Model file for the job. Use its own axes, mm. A direction names the side the tool comes from. Give positions to 0.01 mm unless a question says otherwise; leave off trailing zeros. Order: outer loops, then holes, each group sorted by start corner. A loop starts at its lowest first (then second) coordinate and runs counter-clockwise, first axis right, second up. Notation, with made-up numbers: M -12.5,-15 L 4.5,-15 A14 ccw 4.5,6 Z; hole C 69.5,32.5 d11. An arc over 180 degrees is marked long. Return JSON: item names as keys, results as strings. Group by question number.
1. Slice it at A-A on x = 8. List the corners of the cut face in (y, z), then the cut area to 3 significant figures.
2. Slice it at C-C on y = -5. List the corners of the cut face in (x, z).
3. Pin check, flat tips, straight feed: pin 1 (10 mm diameter, centred on x = -4.5, z = 40, fed in from +Y); pin 2 (3 mm diameter, centred on x = -7.5, z = -39.5, fed in from +Y); pin 3 (8.5 mm diameter, centred on x = -2.5, z = -82.5, fed in from -Y); pin 4 (4 mm diameter, centred on x = -9, z = -42, fed in from +Y). Stop position of each tip, or through.
4. Wall check: probe 1 along Z at (x, y) = (0, 23.25) (3 decimals); probe 2 along Y at (x, z) = (4, 71); probe 3 along X at (y, z) = (21.5, 69.85) (3 decimals). Give the ranges that are in metal, low to high. Write a range as [from, to].
5. 3-axis set-ups, long thin cutter, end or side, ignore diameter. For faces 1 (the face through (10.16, -7, 20)), 2 (the face through (13, -7.62, -39)), 3 (the face through (0, -10.16, -84)), 4 (the face through (-13, 0, -4)): which of +Z, -Z, +X, -X, +Y, -Y reach the whole face in a straight line?
6. Slice it at B-B on z = -35.5. List the corners of the cut face in (x, y), then the cut area to 3 significant figures.
7. Two-plate mould, pull along X, no slides. Class faces 5 (the face through (-15.24, -4, 23)), 6 (the face through (-13, -7.62, -39)), 7 (the face through (0, -16.51, 51)): released by +X, released by -X, zero draft, split by the parting line, or undercut.
8. Slice it at D-D on z = 49. List the corners of the cut face in (x, y), then the cut area to 3 significant figures.
from build123d import *

# Parameters (mm, degrees)
F1_DEPTH     = 16.51
F2_W         = 8.89
F2_H         = 106.68
F3_DEPTH     = 50.8
F4_W         = 5.08
F4_H         = 63.5
F4_W_2       = 25.4
F5_DEPTH     = 5.08
F6_T1_DEPTH  = 5.08
F6_T6_DEPTH  = 43.0474778593
F6_T12_DEPTH = 81.0149557187
F8_DEPTH     = 25.4
F9_W         = 20.32
F9_H         = 15.2493301511
F10_DEPTH    = 2.54
F11_W        = 20.32
F11_H        = 2.54
F12_DEPTH    = 2.54
F13_R        = 0.635
F14_DEPTH    = 2.54
F15_W        = 10.16
F15_H        = 10.16
F15_R        = 0.635
F16_DEPTH    = 1.27


# Not quite as in the source:
# - a fillet or chamfer that OpenCascade refuses, or shapes differently, is made with other operations: its cross-section is extruded or revolved along the edge and cut away or added


with BuildPart() as f1:
    # F0 (on Front) → F1 (new body)
    with BuildSketch(Plane.XZ):
        Polygon((15.24, 6.35), (15.24, 82.55), (10.16, 82.55), (10.16, -82.55), (-10.16, -82.55), (-10.16, 82.55), (-15.24, 82.55), (-15.24, 6.35), (-15.24, -87.63), (15.24, -87.63), align=None)
    extrude(amount=F1_DEPTH)

    # F2 (on face) → F3 (cut)
    with BuildSketch(Plane(origin=(-15.24, 0, 0), x_dir=(0, -1, 0), z_dir=(-1, 0, 0))):
        with Locations((12.065, -34.29)):
            Rectangle(F2_W, F2_H)
    extrude(amount=-F3_DEPTH, mode=Mode.SUBTRACT)

    # F4 (on face) → F5 (join)
    with BuildSketch(Plane.XZ.offset(16.51)):
        with Locations((-12.7, 50.8)):
            Rectangle(F4_W, F4_H)
        with Locations((2.54, 50.8)):
            Rectangle(F4_W_2, F4_H)
    extrude(amount=F5_DEPTH)

    # F6: fillet of radius 15.24 on 1 edges, made by hand

    # F6_s2 → F6_t1 (join)
    with BuildSketch(Plane.YZ.offset(-15.24)):
        with BuildLine():
            ThreePointArc((-21.59, 19.05), (-11.6436636998, 14.1805376301), (-7.62, 3.8630088563))
            Line((-7.62, 3.8630088563), (-7.62, 19.05))
            Line((-7.62, 19.05), (-21.59, 19.05))
        make_face()
    extrude(amount=F6_T1_DEPTH)


with BuildPart() as f6_tool4:
    # F6_s5 → F6_t6 (new body)
    with BuildSketch(Plane.YZ.offset(-15.24)):
        with BuildLine():
            ThreePointArc((-21.59, 19.05), (-11.6436636998, 14.1805376301), (-7.62, 3.8630088563))
            Line((-7.62, 3.8630088563), (-7.62, 19.05))
            Line((-7.62, 19.05), (-21.59, 19.05))
        make_face()
    extrude(amount=F6_T6_DEPTH)

    split(bisect_by=Plane.YZ.offset(15.24), keep=Keep.BOTTOM)

    split(bisect_by=Plane.XZ.offset(16.51), keep=Keep.TOP)


with BuildPart() as f1_1:
    add(f1.part)

    # F6_t3: union F6_tool4
    add(f6_tool4.part)


with BuildPart() as f6_tool10:
    # F6_s11 → F6_t12 (new body)
    with BuildSketch(Plane.YZ.offset(-53.2074778593)):
        with BuildLine():
            ThreePointArc((-21.59, 19.05), (-11.6436636998, 14.1805376301), (-7.62, 3.8630088563))
            Line((-7.62, 3.8630088563), (-7.62, 19.05))
            Line((-7.62, 19.05), (-21.59, 19.05))
        make_face()
    extrude(amount=F6_T12_DEPTH)

    split(bisect_by=Plane.YZ.offset(15.24), keep=Keep.BOTTOM)

    split(bisect_by=Plane.YZ.offset(10.16), keep=Keep.TOP)


with BuildPart() as f1_2:
    add(f1_1.part)

    # F6_t9: union F6_tool10
    add(f6_tool10.part)

    # F7 (on face) → F8 (join)
    with BuildSketch(Plane.XY.offset(82.55)):
        Polygon((10.16, 0), (15.24, 0), (15.24, 22.86), (-15.24, 22.86), (-15.24, 0), (-10.16, 0), align=None)
    extrude(amount=-F8_DEPTH)

    # F9 (on face) → F10 (join)
    with BuildSketch(Plane(origin=(0, 0, 0), x_dir=(-1, 0, 0), z_dir=(0, 1, 0))):
        Polygon((-15.24, -67.3006698489), (-15.24, -87.63), (15.24, -87.63), (15.24, -67.3006698489), (10.16, -67.3006698489), (10.16, -82.55), (-10.16, -82.55), (-10.16, -67.3006698489), align=None)
        with Locations((0, -74.9253349245)):
            Rectangle(F9_W, F9_H)
    extrude(amount=F10_DEPTH)

    # F11 (on face) → F12 (join)
    with BuildSketch(Plane.XZ.offset(7.62)):
        with Locations((0, -81.28)):
            Rectangle(F11_W, F11_H)
        Polygon((-15.24, -80.01), (-15.24, -87.63), (15.24, -87.63), (15.24, -80.01), (10.16, -80.01), (10.16, -82.55), (-10.16, -82.55), (-10.16, -80.01), align=None)
    extrude(amount=F12_DEPTH)

    # F13 (on face) → F14 (cut)
    with BuildSketch(Plane(origin=(0, 22.86, 0), x_dir=(-1, 0, 0), z_dir=(0, 1, 0))):
        with Locations((0, 69.85)):
            Circle(F13_R)
    extrude(amount=-F14_DEPTH, mode=Mode.SUBTRACT)

    # F15 (on face) → F16 (join)
    with BuildSketch(Plane(origin=(0, 22.86, 0), x_dir=(-1, 0, 0), z_dir=(0, 1, 0))):
        with Locations((0, 69.85)):
            Rectangle(F15_W, F15_H)
        with Locations((0, 69.85)):
            Circle(F15_R, mode=Mode.SUBTRACT)
    extrude(amount=F16_DEPTH)


solid = f1_2.part
Result:
{
 "1": {"outline": "M -21.59,19.05 A15.24 cw -16.51,17.72 L -16.51,82.55 L -21.59,82.55 Z; M -10.16,-87.63 L 2.54,-87.63 L 2.54,-67.3 L 0,-67.3 L 0,-82.55 L -7.62,-82.55 L -7.62,-80.01 L -10.16,-80.01 Z; M 0,57.15 L 22.86,57.15 L 22.86,82.55 L 0,82.55 Z", "area": "1,020 mm2"},
 "2": {"outline": "M -15.24,-87.63 L 15.24,-87.63 L 15.24,82.55 L 10.16,82.55 L 10.16,-82.55 L -10.16,-82.55 L -10.16,82.55 L -15.24,82.55 Z"},
 "3": {"pin 1": "stops at y = -16.51", "pin 2": "passes through", "pin 3": "stops at y = -10.16", "pin 4": "stops at y = 0"},
 "4": {"probe 1": "z = [64.77, 69.215], [70.485, 74.93]", "probe 2": "y = [-21.59, -16.51], [0, 24.13]", "probe 3": "x = [-15.24, -0.635], [0.635, 15.24]"},
 "5": {"face 1": "+Z", "face 2": "+X, -X, -Y", "face 3": "-Z, +X, -X, -Y", "face 4": "+X, -X, +Y"},
 "6": {"outline": "M -15.24,-7.62 L -10.16,-7.62 L -10.16,0 L -15.24,0 Z; M 10.16,-7.62 L 15.24,-7.62 L 15.24,0 L 10.16,0 Z", "area": "77.4 mm2"},
 "7": {"face 5": "released by -X", "face 6": "zero draft", "face 7": "undercut"},
 "8": {"outline": "M -15.24,-21.59 L 15.24,-21.59 L 15.24,0 L 10.16,0 L 10.16,-16.51 L -10.16,-16.51 L -10.16,0 L -15.24,0 Z", "area": "323 mm2"}
}
